Input: part model. Units: mm. Frame: model coordinates. A direction names the side the tool comes from. Round coordinates to 2 decimals unless told otherwise and drop trailing zeros. Order: outer loops, then holes, each group sorted by start corner. A loop starts at its lowest first (then second) coordinate and runs counter-clockwise, first axis right, second up. Notation, with made-up numbers: (87.25, 84.5) -> (93.25, 84.5) arc R33 ccw to (93.25, 122.5) -> close; hole circle Ø2 at (-19.75, -5.5). An arc over 180 degrees is marked (long way). Answer as CSV lines item,"result". Start each with the question number.
1) Section query C-C, the plane z = 17. Output: boundary loops of the cut face in (x, y) (1 decimal).
2) Access query for faces 1 (the face through (-6.263, -28.205, 22.003)), 2 (the face through (-40.48, 0.1, 3.13)). Directions: +Z, -Z, +X, -X, +Y, -Y. A direction counts if a zero-diameter tool reaches every point of the face in a straight line with its end or side. Return the directions, or none.
3) Mould query, pull axis Y, two halves, no side actions, for faces 3 (the face through (0, -26, 38.1)), 4 (the face through (5, 0, 6.35)), 5 (the face through (-57.095, 2.513, 3.131)). Classes: +Y half, -Y half, draft (parallel to the pull), parting line (faces both ways), or undercut.
4) Section query D-D, the plane x = 15.5. Output: boundary loops of the cut face in (y, z) (3 decimals), and give its area (3 significant figures).
5) First-contact query: P1, Ø2, axis at y = 23.5, z = 12.5, coming from the -X side; P2, Ø1, axis at x = -13.5, y = -6, coming from the +Z side; P3, Ø1.5, axis at x = -15.5, z = 7, coming from the +Y side; P4, Ø10, axis at x = 34, z = 18, coming from the -Y side. Flat tips, straight axial feed; report the tip coordinate or a pass-through.
6) Section query A-A, the plane y = 0. State how many separate pieces and enclosed holes the cut face has, and give its area (3 significant figures).
7) Line query: L1, parallel to Y at x = 0, z = 3.75 (3 decimals); L2, parallel to Y at x = 0, z = 13.5; L3, parallel to X at y = 35, z = 3.5. Output: solid intervals per line, ascending.
```python
from build123d import *

# Parameters (mm, degrees)
SKETCH1_R        = 57.15
SKETCH1_R_2      = 50.8
EXTRUDE3_DEPTH   = 6.35
SKETCH1_R_3      = 47.625
SKETCH1_R_4      = 28.8925
SKETCH1_R_5      = 2.38125
EXTRUDE3_2_DEPTH = 6.35
SKETCH1_R_6      = 25.4
EXTRUDE3_3_DEPTH = 6.35
SKETCH1_8_R      = 50.8
SKETCH1_8_R_2    = 47.625
EXTRUDE4_DEPTH   = 3.175
SKETCH1_9_R      = 28.8925
SKETCH1_9_R_2    = 25.4
EXTRUDE5_DEPTH   = 38.1


with BuildPart() as part:
    # Sketch1 → Extrude3 (new body)
    with BuildSketch(Plane.XY):
        Circle(SKETCH1_R)
        Circle(SKETCH1_R_2, mode=Mode.SUBTRACT)
    extrude(amount=EXTRUDE3_DEPTH)



with BuildPart() as body_2:
    # Sketch1 → Extrude3 2 (new body)
    with BuildSketch(Plane.XY):
        Circle(SKETCH1_R_3)
        Circle(SKETCH1_R_4, mode=Mode.SUBTRACT)
        with Locations((-38.1, 0)):
            Circle(SKETCH1_R_5, mode=Mode.SUBTRACT)
    extrude(amount=EXTRUDE3_2_DEPTH)


with BuildPart() as body_3:
    # Sketch1 → Extrude3 3 (new body)
    with BuildSketch(Plane.XY):
        Circle(SKETCH1_R_6)
        Circle(SKETCH1_R_5, mode=Mode.SUBTRACT)
    extrude(amount=EXTRUDE3_3_DEPTH)


with BuildPart() as part_1:
    add(part.part)

    add(body_2.part)  # Extrude4 merges body 2
    # Sketch1_8 → Extrude4 (add)
    with BuildSketch(Plane.XY):
        Circle(SKETCH1_8_R)
        Circle(SKETCH1_8_R_2, mode=Mode.SUBTRACT)
    extrude(amount=EXTRUDE4_DEPTH)


    add(body_3.part)  # Extrude5 merges body 3
    # Sketch1_9 → Extrude5 (add)
    with BuildSketch(Plane.XY):
        Circle(SKETCH1_9_R)
        Circle(SKETCH1_9_R_2, mode=Mode.SUBTRACT)
    extrude(amount=EXTRUDE5_DEPTH)


solid = part_1.part
```
Findings:
1,outline,"circle Ø57.8 at (0, 0); hole circle Ø50.8 at (0, 0)"
2,face 1,"+Z"
2,face 2,"+Z, -Z"
3,face 3,"draft"
3,face 4,"undercut"
3,face 5,"parting line"
4,outline,"(-55.008, 0) -> (55.008, 0) -> (55.008, 6.35) -> (48.378, 6.35) -> (48.378, 3.175) -> (45.032, 3.175) -> (45.032, 6.35) -> (24.383, 6.35) -> (24.383, 38.1) -> (20.122, 38.1) -> (20.122, 6.35) -> (-20.122, 6.35) -> (-20.122, 38.1) -> (-24.383, 38.1) -> (-24.383, 6.35) -> (-45.032, 6.35) -> (-45.032, 3.175) -> (-48.378, 3.175) -> (-48.378, 6.35) -> (-55.008, 6.35) -> close"
4,area,"948 mm^2"
5,P1,"stops at x = -18.13"
5,P2,"stops at z = 6.35"
5,P3,"stops at y = 55.11"
5,P4,"passes through"
6,separate pieces,"3"
6,enclosed holes,"0"
6,area,"867 mm^2"
7,L1,"y = -57.15 to -50.8, -47.625 to -2.381, 2.381 to 47.625, 50.8 to 57.15"
7,L2,"y = -28.89 to -25.4, 25.4 to 28.89"
7,L3,"x = -45.18 to -36.82, -32.3 to 32.3, 36.82 to 45.18"
